```python
from build123d import *

# Parameters (mm, degrees)
F0_R     = 4
F1_DEPTH = 12
F2_R     = 7
F3_DEPTH = 5
F5_DEPTH = 4.5
F6_R     = 3.135896
F7_DEPTH = 25


with BuildPart() as f1:
    # F0 (on Top) → F1 (new body)
    with BuildSketch(Plane.XY):
        Circle(F0_R)
    extrude(amount=F1_DEPTH)

    # F2 (on face) → F3 (join)
    with BuildSketch(Plane.XY.offset(12)):
        Circle(F2_R)
    extrude(amount=F3_DEPTH)

    # F4 (on face) → F5 (cut)
    with BuildSketch(Plane.XY.offset(17)):
        Polygon((5.887997, -0.107183), (3.036822, 5.045564), (-2.851175, 5.152747), (-5.887997, 0.107183), (-3.036822, -5.045564), (2.851175, -5.152747), align=None)
    extrude(amount=-F5_DEPTH, mode=Mode.SUBTRACT)

    # F6 (on face) → F7 (cut)
    with BuildSketch(Plane(origin=(0, 0, 0), x_dir=(1, 0, 0), z_dir=(0, 0, -1))):
        Circle(F6_R)
    extrude(amount=-F7_DEPTH, mode=Mode.SUBTRACT)


solid = f1.part
```
Design review of the part built by this model. Coordinates are the model's own, in mm. A direction names the side the tool comes from. Round coordinates to 2 decimals unless told otherwise and drop trailing zeros. Order: outer loops, then holes, each group sorted by start corner. A loop starts at its lowest first (then second) coordinate and runs counter-clockwise, first axis right, second up. Notation, with made-up numbers: (33, 77.25) - (59, 77.25) arc R21 ccw to (59, 83.25) - close; hole circle Ø7 at (-32.5, 40.5). An arc over 180 degrees is marked (long way). Return JSON: item names as keys, results as strings.
Q1. Machinability: for faces 4 (the flat face through (-5, -2, 17)), 5 (the flat face through (3, -3, 12)), 6 (the flat face through (-4.348, 2.665, 14.782)), which of the approach directions +Z, -Z, +X, -X, +Y, -Y give a long, thin tool a straight path to every point of the face, cutting with its end or side? Answer none if there is none.
Computed values:
{"face 4": "+Z, +X, -X, +Y, -Y", "face 5": "-Z", "face 6": "+Z"}
Q2. Consider section C-C on y = -0.5. Write out the cut boundary in (x, z).
Computed values:
{"outline": "(-6.98, 12) - (-3.97, 12) - (-3.97, 0) - (-3.1, 0) - (-3.1, 12.5) - (-5.55, 12.5) - (-5.55, 17) - (-6.98, 17) - close; (3.1, 0) - (3.97, 0) - (3.97, 12) - (6.98, 12) - (6.98, 17) - (5.65, 17) - (5.65, 12.5) - (3.1, 12.5) - close"}
Q3. Consider section D-D on x = -4.5. Write out the cut boundary in (y, z), plus the area to 3 significant figures.
Computed values:
{"outline": "(-5.36, 12) - (5.36, 12) - (5.36, 17) - (2.41, 17) - (2.41, 12.5) - (-2.4, 12.5) - (-2.4, 17) - (-5.36, 17) - close", "area": "32.0 mm2"}
Q4. The part is to be moulded in two halves that separate along X. For faces 1 (the flat face through (2, -3, 0)), 2 (the cylindrical face through (6.466, -2.681, 14.465)), 3 (the flat face through (3, 2, 12.5)), say which applies: pulls with the +X half, pulls with the -X half, needs draft (parallel to the pull), parting line crosses it, or undercut.
Computed values:
{"face 1": "needs draft", "face 2": "parting line crosses it", "face 3": "undercut"}
Q5. Wall thickness on L1, parallel to Y at x = 0, z = 5; L2, parallel to Z at x = -3.25, y = 1.75; L3, parallel to Z at x = -1, y = -5.75: over which ranges is each line inside the solid? List them lowest first. Write a range as [from, to].
Computed values:
{"L1": "y = [-4, -3.14], [3.14, 4]", "L2": "z = [0, 12.5]", "L3": "z = [12, 17]"}
Q6. Consider section B-B on x = 0. Write out the cut boundary in (y, z).
Computed values:
{"outline": "(-7, 12) - (-4, 12) - (-4, 0) - (-3.14, 0) - (-3.14, 12.5) - (-5.1, 12.5) - (-5.1, 17) - (-7, 17) - close; (3.14, 0) - (4, 0) - (4, 12) - (7, 12) - (7, 17) - (5.1, 17) - (5.1, 12.5) - (3.14, 12.5) - close"}
Q7. For pin 1 Ø3 at (x, z) = (4, 14.5) entering from -Y; pin 2 Ø4 at (y, z) = (-5, 14.5) entering from +X; pin 3 Ø7 at (x, y) = (0, 0) entering from +Z; pin 4 Ø8 at (y, z) = (0, 9.5) entering from +X, all flat-tipped, find the tip position at first contact; note any pin that passes through.
Computed values:
{"pin 1": "stops at y = -6.54", "pin 2": "stops at x = 6.32", "pin 3": "stops at z = 12.5", "pin 4": "stops at x = 7"}
Q8. Consider section A-A on z = 16.25. Write out the cut boundary in (x, y), plus the area to 3 significant figures.
Computed values:
{"outline": "circle Ø14 at (0, 0); hole (-5.89, 0.11) - (-3.04, -5.05) - (2.85, -5.15) - (5.89, -0.11) - (3.04, 5.05) - (-2.85, 5.15) - close", "area": "63.8 mm2"}
